The listing builds one solid part. Answer for the finished solid, in the listing's coordinates (mm). A direction names the side the tool comes from. Give positions to 0.01 mm unless a question says otherwise; leave off trailing zeros. Write each loop counter-clockwise with the first axis right and the second up, starting at its lowest first coordinate (ties: lowest second). Pieces come first, ordered by that corner, then holes. Notation, with made-up numbers: M 35,17.25 L 50,17.25 A34 ccw 50,47.25 Z; hole C 37.25,26 d11. An arc over 180 degrees is marked long. Return JSON: item names as keys, results as strings.
from build123d import *

# Parameters (mm, degrees)
SKETCH_1_W                  = 12
SKETCH_1_H                  = 1.2
SKETCH_2_R                  = 6.25
EXTRUDE_1_DEPTH             = 0.1
SKETCH_3_R                  = 2.5
EXTRUDE_2_DEPTH             = 4
EXTRUDE_START               = 16.9
SKETCH_5_R                  = 6.25
EXTRUDE_4_DEPTH             = 16.9
HOLE_WIZARD_3_2_3_2_1_D     = 3.2
HOLE_WIZARD_3_2_3_2_1_DEPTH = 18.1


with BuildPart() as part:
    # 草图1 → 旋转1 (revolve)
    with BuildSketch(Plane.XY, mode=Mode.PRIVATE) as revolve_1_sk:
        with Locations((6, 17.5)):
            Rectangle(SKETCH_1_W, SKETCH_1_H)
    revolve(revolve_1_sk.sketch.rotate(Axis((0, 18.1, 0), (0, -1, 0)), 270), axis=Axis((0, 18.1, 0), (0, -1, 0)))

    # 草图2 → 凸台-拉伸1 (add)
    with BuildSketch(Plane(origin=(0, 18.1, 0), x_dir=(-1, 0, 0), z_dir=(0, 1, 0))):
        with Locations(Location((0, 0, 0), (0, 0, 90))):
            Circle(SKETCH_2_R)
    extrude(amount=EXTRUDE_1_DEPTH)

    # 草图3 → 凸台-拉伸2 (add)
    with BuildSketch(Plane(origin=(0, 18.2, 0), x_dir=(-1, 0, 0), z_dir=(0, 1, 0))):
        with Locations(Location((0, 0, 0), (0, 0, 90))):
            Circle(SKETCH_3_R)
    extrude(amount=EXTRUDE_2_DEPTH)

    # 草图5 → 凸台-拉伸4 (add)
    with BuildSketch(Plane.XZ.offset(-16.9).offset(EXTRUDE_START)):
        with Locations(Location((0, 0, 0), (0, 0, 90))):
            Circle(SKETCH_5_R)
    extrude(amount=-EXTRUDE_4_DEPTH)

    # Ø3.2 (3.2) 直径孔1
    with Locations(Plane(origin=(0, 18.1, 0), x_dir=(1, 0, 0), z_dir=(0, 1, 0))):
        with Locations((-7.794228634, -4.5), (7.794228634, -4.5), (0, 9)):
            Hole(HOLE_WIZARD_3_2_3_2_1_D / 2, depth=HOLE_WIZARD_3_2_3_2_1_DEPTH)


solid = part.part
Item 1: Determine the mould class of faces 1 (the flat face through (0, 22.2, 0)), 2 (the cylindrical face through (9.064, 17.492, 5.474)), 3 (the cylindrical face through (3.604, 17.508, -11.446)) for opening direction X: +X half, -X half, draft (parallel to the pull), parting line (faces both ways), or undercut.
Geometry results:
{"face 1": "draft", "face 2": "undercut", "face 3": "parting line"}
Item 2: Given pin 1 Ø4 at (x, z) = (-7.79, 4.5) entering from +Y; pin 2 Ø12 at (x, z) = (4, -5) entering from +Y; pin 3 Ø5 at (y, z) = (9.5, 0.5) entering from -X; pin 4 Ø2 at (y, z) = (11.5, -3.5) entering from +X, each flat-ended and moving along its own axis, determine where each tip first touches the part or whether it passes through.
Geometry results:
{"pin 1": "stops at y = 18.1", "pin 2": "stops at y = 22.2", "pin 3": "stops at x = -6.25", "pin 4": "stops at x = 5.73"}
Item 3: Find the intervals of material crossed by line 1 (X direction, y = 17.5, z = 4.5); line 2 (Y direction, x = -3.75, z = 8.75); line 3 (X direction, y = 17.5, z = -9), in increasing order.
Geometry results:
{"line 1": "x = -11.12 to -9.39, -6.19 to 6.19, 9.39 to 11.12", "line 2": "y = 16.9 to 18.1", "line 3": "x = -7.94 to -1.6, 1.6 to 7.94"}
Item 4: A cutting plane is placed at A-A, the plane x = 0. Write down the section's boundary in (y, z), plus the area to 3 significant figures.
Geometry results:
{"outline": "M 0,-6.25 L 16.9,-6.25 L 16.9,-7.4 L 18.1,-7.4 L 18.1,-6.25 L 18.2,-6.25 L 18.2,-2.5 L 22.2,-2.5 L 22.2,2.5 L 18.2,2.5 L 18.2,6.25 L 18.1,6.25 L 18.1,12 L 16.9,12 L 16.9,6.25 L 0,6.25 Z; M 16.9,-12 L 18.1,-12 L 18.1,-10.6 L 16.9,-10.6 Z", "area": "257 mm2"}
Item 5: A cutting plane is placed at C-C, the plane z = 4.5. Write down the section's boundary in (x, y).
Geometry results:
{"outline": "M -11.12,16.9 L -9.39,16.9 L -9.39,18.1 L -11.12,18.1 Z; M -6.19,16.9 L -4.34,16.9 L -4.34,0 L 4.34,0 L 4.34,16.9 L 6.19,16.9 L 6.19,18.1 L 4.34,18.1 L 4.34,18.2 L -4.34,18.2 L -4.34,18.1 L -6.19,18.1 Z; M 9.39,16.9 L 11.12,16.9 L 11.12,18.1 L 9.39,18.1 Z"}
Item 6: A cutting plane is placed at D-D, the plane x = -9. Write down the section's boundary in (y, z).
Geometry results:
{"outline": "M 16.9,-7.94 L 18.1,-7.94 L 18.1,3.45 L 16.9,3.45 Z; M 16.9,5.55 L 18.1,5.55 L 18.1,7.94 L 16.9,7.94 Z"}
Item 7: Which of the six approach directions +Z, -Z, +X, -X, +Y, -Y give full straight-line access (tool end or side, diameter ignored) to faces 4 (the cylindrical face through (0.35, 17.49, -7.44)), 5 (the flat face through (-5, 16.9, 5)), 6 (the flat face through (-3, 18.2, 0))?
Geometry results:
{"face 4": "+Y, -Y", "face 5": "-Y", "face 6": "+Y"}
Item 8: A cutting plane is placed at B-B, the plane z = -10. Write down the section's boundary in (x, y).
Geometry results:
{"outline": "M -6.63,16.9 L -1.25,16.9 L -1.25,18.1 L -6.63,18.1 Z; M 1.25,16.9 L 6.63,16.9 L 6.63,18.1 L 1.25,18.1 Z"}
